Build history of the part. All positions in model axes, mm. Face numbers are marked on the shaded views. A direction names the side the tool comes from. Round coordinates to 2 decimals unless told otherwise and drop trailing zeros. Write each loop counter-clockwise with the first axis right and the second up, starting at its lowest first coordinate (ties: lowest second). Pieces come first, ordered by that corner, then holes. Notation, with made-up numbers: (53.5, -14) - (93.5, -14) arc R5 ccw to (93.5, -7) - close; hole circle Ø3 at (64, 5). An arc over 180 degrees is marked (long way). Answer as a JSON object with one key per item and string values. Group by question number.
Item 1: Slice it at D-D, the plane y = 8. List the corners of the cut face in (x, z), then the cut area to 3 significant figures.
Item 2: Probe line 1 (Y direction, x = -28.5, z = 6); line 2 (X direction, y = 35, z = 5.25); line 3 (Y direction, x = -8.5, z = 5.25). List the from-to ranges inside material, lowest first. Write a range as from..to.
Item 3: Slice it at B-B, the plane x = -8.5. List the corners of the cut face in (y, z) (3 decimals).
Item 4: Two-plate mould, pull along Z, no slides. Class the marked faces 3, 4 and 5: +Z half, -Z half, draft (parallel to the pull), parting line (faces both ways), or undercut.
Item 5: Which spindle directions (+Z, -Z, +X, -X, +Y, -Y) get a long thin tool onto all of the face, cutting with end or side? Do the marked faces 1 and 2. Say none if no direction does.
Item 6: Slice it at C-C, the plane z = 11.25. List the corners of the cut face in (x, y).
Item 7: Flat gauge pins, fed straight in: pin 1 (1 mm diameter, centred on x = -16.5, z = -2.5, fed in from +Y); pin 2 (2.5 mm diameter, centred on x = -28.5, y = 39, fed in from +Z); pin 3 (20 mm diameter, centred on x = -25, y = 72, fed in from +Z); pin 4 (10 mm diameter, centred on x = -13, y = 79, fed in from -Z) (3 decimals). Where does each tip first touch, or does it go through?
Item 8: Slice it at A-A, the plane y = 35. List the corners of the cut face in (x, z), then the cut area to 3 significant figures.
from build123d import *

# Parameters (mm, degrees)
SKETCH1_W                            = 35
SKETCH1_H                            = 60
BOSS_EXTRUDE1_DEPTH                  = 15
SKETCH2_R                            = 1.5
SKETCH2_R_2                          = 0.95
CUT_EXTRUDE1_DEPTH                   = 72.063352018
MIRROR1_OUTLINE_R                    = 0.95
MIRROR1_DEPTH                        = 15
SKETCH3_R                            = 8
BOSS_EXTRUDE2_DEPTH                  = 12
SKETCH4_R                            = 6.5
CUT_EXTRUDE2_DEPTH                   = 72.063352018
SKETCH5_W                            = 35
SKETCH5_H                            = 5
BOSS_EXTRUDE4_DEPTH                  = 5
BOSS_EXTRUDE4_DIRECTION_2_REACH      = 73.063
BOSS_EXTRUDE4_DIRECTION_2_END_RADIUS = 8
BOSS_EXTRUDE7_DEPTH                  = 35


# Read off the part's stored shape, not the designer's step: Mirror1
with BuildPart() as part:
    # Sketch1 → Boss-Extrude1 (new body)
    with BuildSketch(Plane.XY):
        with Locations((-17.5, 30)):
            Rectangle(SKETCH1_W, SKETCH1_H)
    extrude(amount=BOSS_EXTRUDE1_DEPTH)

    # Sketch2 → Cut-Extrude1 (cut, through all)
    with BuildSketch(Plane.XY.offset(15)):
        with Locations((-28.5, 8)):
            Circle(SKETCH2_R)
        with Locations((-26.5, 13)):
            Circle(SKETCH2_R_2)
        with Locations((-26.5, 35)):
            Circle(SKETCH2_R_2)
        with Locations((-28.5, 39)):
            Circle(SKETCH2_R)
    extrude(amount=-CUT_EXTRUDE1_DEPTH, mode=Mode.SUBTRACT)

    # Mirror1 outline → Mirror1 (cut)
    with BuildSketch(Plane.XY):
        with Locations((-8.5, 35)):
            Circle(MIRROR1_OUTLINE_R)
        with Locations((-8.5, 13)):
            Circle(MIRROR1_OUTLINE_R)
    extrude(amount=MIRROR1_DEPTH, mode=Mode.SUBTRACT)

    # Sketch3 → Boss-Extrude2 (add)
    with BuildSketch(Plane.ZY.offset(35)):
        with Locations((-4, 50)):
            Circle(SKETCH3_R)
    boss_extrude2 = extrude(amount=-BOSS_EXTRUDE2_DEPTH)

    # Sketch4 → Cut-Extrude2 (cut, through all)
    with BuildSketch(Plane.ZY.offset(35)):
        with Locations(Location((-4, 50, 0), (0, 0, 270))):
            Circle(SKETCH4_R)
    cut_extrude2 = extrude(amount=-CUT_EXTRUDE2_DEPTH, mode=Mode.SUBTRACT)

    # Mirror2: Boss-Extrude2, Cut-Extrude2 across plane
    add(boss_extrude2.mirror(Plane(origin=(-17.5, 0, 0), x_dir=(0, 0, 1), z_dir=(1, 0, 0))))
    add(cut_extrude2.mirror(Plane(origin=(-17.5, 0, 0), x_dir=(0, 0, 1), z_dir=(1, 0, 0))), mode=Mode.SUBTRACT)

    # Sketch5 → Boss-Extrude4 (add)
    with BuildSketch(Plane(origin=(0, 60, 0), x_dir=(1, 0, 0), z_dir=(0, 1, 0))):
        with Locations((-17.5, 0)):
            Rectangle(SKETCH5_W, SKETCH5_H)
    extrude(amount=BOSS_EXTRUDE4_DEPTH)

    # Boss-Extrude4 direction 2: up to this cylinder (the profile starts outside it)
    boss_extrude4_direction_2_end = Plane(origin=(-17.5, 50, -4), z_dir=(-1, 0, 0)) * Cylinder(BOSS_EXTRUDE4_DIRECTION_2_END_RADIUS, 163.126, mode=Mode.PRIVATE)
    # Sketch5 → Boss-Extrude4 direction 2 (add, up to the surface)
    with BuildSketch(Plane(origin=(0, 60, 0), x_dir=(1, 0, 0), z_dir=(0, 1, 0)), mode=Mode.PRIVATE) as boss_extrude4_direction_2_sk1:
        with Locations((-17.5, 0)):
            Rectangle(SKETCH5_W, SKETCH5_H)
    boss_extrude4_direction_2_tool1 = extrude(boss_extrude4_direction_2_sk1.sketch, amount=-BOSS_EXTRUDE4_DIRECTION_2_REACH, mode=Mode.PRIVATE) - boss_extrude4_direction_2_end
    add(boss_extrude4_direction_2_tool1.solids().sort_by_distance((-17.5, 60, 0))[0])

    # Sketch12 → Boss-Extrude7 (add, through all)
    with BuildSketch(Plane.ZY.offset(35)):
        Polygon((-2.5, 65), (-7.175, 65), (-7.175, 90), (-11.175, 90), (-11.175, 60), (-2.5, 60), align=None)
    extrude(amount=-BOSS_EXTRUDE7_DEPTH)


solid = part.part
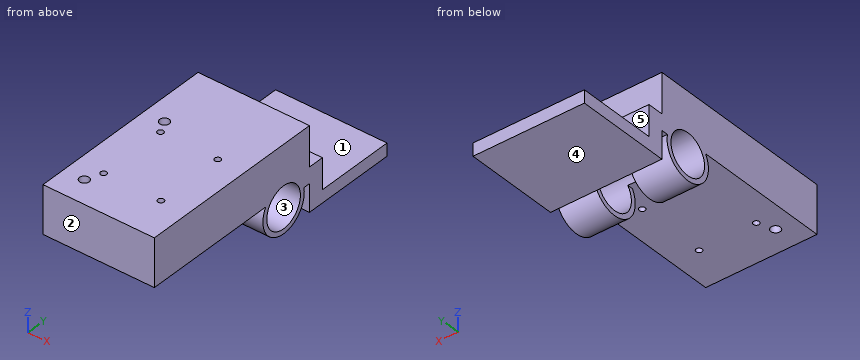
Geometry says:
{
 "1": {"outline": "(-35, 0) - (-30, 0) - (-30, 15) - (-35, 15) - close; (-27, 0) - (0, 0) - (0, 15) - (-27, 15) - close", "area": "480 mm^2"},
 "2": {"line 1": "y = 0..6.5, 9.5..37.5, 40.5..60", "line 2": "x = -35..-27.45, -25.55..-9.45, -7.55..0", "line 3": "y = 0..12.05, 13.95..34.05, 35.95..60"},
 "3": {"outline": "(0, 0) - (12.05, 0) - (12.05, 15) - (0, 15) - close; (13.95, 0) - (34.05, 0) - (34.05, 15) - (13.95, 15) - close; (35.95, 0) - (43.072, 0) arc R8 ccw (long way) to (57.858, -2.5) - (60, -2.5) - (60, -11.175) - (90, -11.175) - (90, -7.175) - (65, -7.175) - (65, 2.5) - (60, 2.5) - (60, 15) - (35.95, 15) - close; hole circle Ø13 at (50, -4)"},
 "4": {"face 3": "undercut", "face 4": "-Z half", "face 5": "draft"},
 "5": {"face 1": "+Z, +X, -X, +Y", "face 2": "+Z, -Z, +X, -X, -Y"},
 "6": {"outline": "(-35, 0) - (0, 0) - (0, 60) - (-35, 60) - close; hole circle Ø3 at (-28.5, 8); hole circle Ø3 at (-28.5, 39); hole circle Ø1.9 at (-26.5, 13); hole circle Ø1.9 at (-26.5, 35); hole circle Ø1.9 at (-8.5, 13); hole circle Ø1.9 at (-8.5, 35)"},
 "7": {"pin 1": "stops at y = 65", "pin 2": "passes through", "pin 3": "stops at z = 2.5", "pin 4": "stops at z = -11.175"},
 "8": {"outline": "(-35, 0) - (-27.45, 0) - (-27.45, 15) - (-35, 15) - close; (-25.55, 0) - (-9.45, 0) - (-9.45, 15) - (-25.55, 15) - close; (-7.55, 0) - (0, 0) - (0, 15) - (-7.55, 15) - close", "area": "468 mm^2"}
}
